from build123d import *

# Parameters (mm, degrees)
SKETCH1_W               = 22
SKETCH1_H               = 74
BOSS_EXTRUDE1_DEPTH     = 330
SKETCH4_W               = 10
SKETCH4_H               = 62
CUT_EXTRUDE2_DEPTH      = 1
CUT_EXTRUDE2_DEPTH_BACK = 331
SKETCH6_W               = 22
SKETCH6_H               = 74
SKETCH6_W_2             = 20
SKETCH6_H_2             = 72
CUT_EXTRUDE4_DEPTH      = 107
SKETCH7_W               = 22
SKETCH7_H               = 74
SKETCH7_W_2             = 20
SKETCH7_H_2             = 72
CUT_EXTRUDE5_DEPTH      = 107
FILLET1_R               = 3
FILLET2_R               = 4


with BuildPart() as part:
    # Sketch1 → Boss-Extrude1 (new body)
    with BuildSketch(Plane.XY):
        Rectangle(SKETCH1_W, SKETCH1_H)
    extrude(amount=BOSS_EXTRUDE1_DEPTH)

    # Sketch4 → Cut-Extrude2 (cut, two sides)
    with BuildSketch(Plane.XY.offset(330)) as cut_extrude2_sk:
        Rectangle(SKETCH4_W, SKETCH4_H)
    extrude(amount=CUT_EXTRUDE2_DEPTH, mode=Mode.SUBTRACT)
    extrude(cut_extrude2_sk.sketch, amount=-CUT_EXTRUDE2_DEPTH_BACK, mode=Mode.SUBTRACT)

    # Sketch6 → Cut-Extrude4 (cut)
    with BuildSketch(Plane.XY.offset(330)):
        Rectangle(SKETCH6_W, SKETCH6_H)
        Rectangle(SKETCH6_W_2, SKETCH6_H_2, mode=Mode.SUBTRACT)
    extrude(amount=-CUT_EXTRUDE4_DEPTH, mode=Mode.SUBTRACT)

    # Sketch7 → Cut-Extrude5 (cut)
    with BuildSketch(Plane(origin=(0, 0, 0), x_dir=(-1, 0, 0), z_dir=(0, 0, -1))):
        Rectangle(SKETCH7_W, SKETCH7_H)
        Rectangle(SKETCH7_W_2, SKETCH7_H_2, mode=Mode.SUBTRACT)
    extrude(amount=-CUT_EXTRUDE5_DEPTH, mode=Mode.SUBTRACT)

    # Fillet1
    fillet1_edges = [part.edges().sort_by_distance(p)[0] for p in [
        (10, -36, 276.5),
        (-10, -36, 276.5),
        (-10, 36, 276.5),
        (10, 36, 276.5),
        (-10, -36, 53.5),
        (10, -36, 53.5),
        (10, 36, 53.5),
        (-10, 36, 53.5),
    ]]
    fillet(fillet1_edges, radius=FILLET1_R)

    # Fillet2
    fillet2_edges = [part.edges().sort_by_distance(p)[0] for p in [
        (11, -37, 165),
        (-11, -37, 165),
        (-11, 37, 165),
        (11, 37, 165),
    ]]
    fillet(fillet2_edges, radius=FILLET2_R)


solid = part.part
Could you check a few things on this model? Use its own coordinates, in mm. A direction names the side the tool comes from. Give positions to 0.01 mm unless a question says otherwise; leave off trailing zeros. Loops run counter-clockwise (first coordinate to the right, second up) from the corner with the lowest first, then second, coordinate; pieces in that order, holes last. Notation, with made-up numbers: (67, -5) -> (94, -5) arc R18 cw to (94, 2) -> close; hole circle Ø8 at (37.25, -37). An arc over 180 degrees is marked (long way). Answer as CSV lines item,"result". Start each with the question number.
(1) If we section it at D-D on z = 42: Write out the boundary of the cut face in (x, y), then the cut area to 3 significant figures.
(2) I'm going to push flat-ended pins straight in: pin 1 Ø10 at (y, z) = (6, 293) entering from +X; pin 2 Ø3 at (x, z) = (-1, 236) entering from +Y; pin 3 Ø10 at (y, z) = (-13.5, 89.5) entering from -X. Where does each tip first touch, or does it pass through?
(3) I need wall thicknesses on probe 1 along X at (y, z) = (-15, 142.5); probe 2 along Y at (x, z) = (1, 73); probe 3 along Y at (x, z) = (-3, 112.5). Which ranges of each line are inside material? Lowest first, please.
(4) We'd pull the mould along X, two halves only. Please class faces 1 (the flat face through (-5, 0, 167)), 2 (the flat face through (11, 0, 164)), 3 (the flat face through (0, 36, 277)), 4 (the flat face through (-10, 0, 277)): released by +X, released by -X, zero draft, split by the parting line, or undercut.
(5) If we section it at B-B on y = 14: Write out the boundary of the cut face in (x, z), then the cut area to 3 significant figures.
(6) If we section it at A-A on z = 175.5: Write out the boundary of the cut face in (x, y), then the cut area to 3 significant figures.
(7) Which directions (+Z, -Z, +X, -X, +Y, -Y) give clear straight access to the entire face, cutting with the end or side of a thin tool? Please do faces 5 (the flat face through (5, 0, 167)), 6 (the flat face through (0, -36, 53)), 7 (the flat face through (10, 0, 53)).
(8) If we section it at C-C on x = 1: Write out the boundary of the cut face in (y, z).
Computed:
1,outline,"(-10, -33) arc R3 ccw to (-7, -36) -> (7, -36) arc R3 ccw to (10, -33) -> (10, 33) arc R3 ccw to (7, 36) -> (-7, 36) arc R3 ccw to (-10, 33) -> close; hole (-5, -31) -> (5, -31) -> (5, 31) -> (-5, 31) -> close"
1,area,"812 mm2"
2,pin 1,"stops at x = 10"
2,pin 2,"stops at y = 36"
2,pin 3,"stops at x = -10"
3,probe 1,"x = -11 to -5, 5 to 11"
3,probe 2,"y = -36 to -31, 31 to 36"
3,probe 3,"y = -37 to -31, 31 to 37"
4,face 1,"undercut"
4,face 2,"released by +X"
4,face 3,"zero draft"
4,face 4,"released by -X"
5,outline,"(-11, 107) -> (-10, 107) -> (-10, 0) -> (-5, 0) -> (-5, 330) -> (-10, 330) -> (-10, 223) -> (-11, 223) -> close; (5, 0) -> (10, 0) -> (10, 107) -> (11, 107) -> (11, 223) -> (10, 223) -> (10, 330) -> (5, 330) -> close"
5,area,"3,530 mm2"
6,outline,"(-11, -33) arc R4 ccw to (-7, -37) -> (7, -37) arc R4 ccw to (11, -33) -> (11, 33) arc R4 ccw to (7, 37) -> (-7, 37) arc R4 ccw to (-11, 33) -> close; hole (-5, -31) -> (5, -31) -> (5, 31) -> (-5, 31) -> close"
6,area,"994 mm2"
7,face 5,"+Z, -Z"
7,face 6,"-Z, +X, -X, -Y"
7,face 7,"-Z, +X, +Y, -Y"
8,outline,"(-37, 107) -> (-36, 107) -> (-36, 0) -> (-31, 0) -> (-31, 330) -> (-36, 330) -> (-36, 223) -> (-37, 223) -> close; (31, 0) -> (36, 0) -> (36, 107) -> (37, 107) -> (37, 223) -> (36, 223) -> (36, 330) -> (31, 330) -> close"
